```python
from build123d import *

# Parameters (mm, degrees)
BOSS_EXTRUDE1_START     = -38.1
SKETCH1_R               = 14.2875
SKETCH1_R_2             = 3.175
SKETCH1_R_3             = 3.2639
BOSS_EXTRUDE1_DEPTH     = 9.525
CUT_EXTRUDE1_REACH      = 194.229
CUT_EXTRUDE1_END_RADIUS = 14.2875
SKETCH2_R               = 2.6035
FILLET1_R               = 6.35


with BuildPart() as part:
    # Sketch1 → Boss-Extrude1 (new body)
    with BuildSketch(Plane(origin=(0, 0, 0), x_dir=(0, 0, -1), z_dir=(1, 0, 0)).offset(BOSS_EXTRUDE1_START)):
        with BuildLine():
            Line((-42.525623825, 632.652514423), (-55.415953018, 737.356140976))
            Line((-55.415953018, 737.356140976), (-55.415953018, 788.156140976))
            Line((-55.415953018, 788.156140976), (20.784046982, 788.156140976))
            Line((20.784046982, 788.156140976), (20.784046982, 737.356140976))
            Line((20.784046982, 737.356140976), (7.89371779, 632.652514423))
            ThreePointArc((7.89371779, 632.652514423), (-17.315953018, 610.356140976), (-42.525623825, 632.652514423))
        make_face()
        with Locations((-17.315953018, 635.756140976)):
            Circle(SKETCH1_R, mode=Mode.SUBTRACT)
        with Locations((-45.890953018, 775.456140976)):
            Circle(SKETCH1_R_2, mode=Mode.SUBTRACT)
        with Locations((-17.315953018, 762.756140976)):
            Circle(SKETCH1_R_2, mode=Mode.SUBTRACT)
        with Locations((-45.890953018, 750.056140976)):
            Circle(SKETCH1_R_2, mode=Mode.SUBTRACT)
        with Locations((11.259046982, 750.056140976)):
            Circle(SKETCH1_R_2, mode=Mode.SUBTRACT)
        with Locations((11.259046982, 775.456140976)):
            Circle(SKETCH1_R_2, mode=Mode.SUBTRACT)
        with Locations((8.084046982, 696.081140976)):
            Circle(SKETCH1_R_3, mode=Mode.SUBTRACT)
        with Locations((-17.315953018, 680.206140976)):
            Circle(SKETCH1_R_2, mode=Mode.SUBTRACT)
        with Locations((-42.715953018, 696.081140976)):
            Circle(SKETCH1_R_3, mode=Mode.SUBTRACT)
    extrude(amount=-BOSS_EXTRUDE1_DEPTH)

    # Cut-Extrude1: up to this cylinder (the profile starts outside it)
    cut_extrude1_end = Plane(origin=(-42.8625, 635.756140976, 17.315953018), z_dir=(1, 0, 0)) * Cylinder(CUT_EXTRUDE1_END_RADIUS, 418.033, mode=Mode.PRIVATE)
    # Sketch2 → Cut-Extrude1 (cut, up to the surface)
    with BuildSketch(Plane(origin=(0, 610.356140976, 0), x_dir=(-1, 0, 0), z_dir=(0, -1, 0)), mode=Mode.PRIVATE) as cut_extrude1_sk1:
        with Locations(Location((42.8625, -17.315953018, 0), (0, 0, 90))):
            Circle(SKETCH2_R)
    cut_extrude1_tool1 = extrude(cut_extrude1_sk1.sketch, amount=-CUT_EXTRUDE1_REACH, mode=Mode.PRIVATE) - cut_extrude1_end
    add(cut_extrude1_tool1.solids().sort_by_distance((-42.8625, 610.356141, 17.315953))[0], mode=Mode.SUBTRACT)

    # Fillet1
    fillet1_edges = [part.edges().sort_by_distance(p)[0] for p in [
        (-42.8625, 737.356140976, 55.415953018),
        (-42.8625, 788.156140976, 55.415953018),
        (-42.8625, 788.156140976, -20.784046982),
        (-42.8625, 737.356140976, -20.784046982),
    ]]
    fillet(fillet1_edges, radius=FILLET1_R)


solid = part.part
```
The model under review builds one solid part; all positions refer to its coordinate system, in mm. Give positions to 0.01 mm unless a question says otherwise; leave off trailing zeros. Write each loop counter-clockwise with the first axis right and the second up, starting at its lowest first coordinate (ties: lowest second). Pieces come first, ordered by that corner, then holes. Notation, with made-up numbers: (-4, -7.5) -> (29, -7.5) arc R31 cw to (29, 16.5) -> close; hole circle Ø2 at (34, 3.25). An arc over 180 degrees is marked (long way). Put each result on its own line as item: value.
(1) For pin 1 Ø8.5 at (y, z) = (775.46, 45.89) entering from +X; pin 2 Ø2 at (x, y) = (-42.5, 686.5) entering from -Z, all flat-tipped, find the tip position at first contact; note any pin that passes through.
Results are:
pin 1: x = -38.1
pin 2: z = -14.65
(2) We need section B-B, the plane z = 27. Give the boundary of the cut face in (x, y) (3 decimals).
Results are:
outline: (-47.625, 612.275) -> (-38.1, 612.275) -> (-38.1, 625.251) -> (-47.625, 625.251) -> close; (-47.625, 646.261) -> (-38.1, 646.261) -> (-38.1, 788.156) -> (-47.625, 788.156) -> close
(3) We need section C-C, the plane y = 729.5. Give the boundary of the cut face in (x, z) (3 decimals), and give its area (3 significant figures).
Results are:
outline: (-47.625, -19.817) -> (-38.1, -19.817) -> (-38.1, 54.449) -> (-47.625, 54.449) -> close
area: 707 mm²
(4) We need section A-A, the plane z = 10. Give the boundary of the cut face in (x, y) (3 decimals), and give its area (3 significant figures).
Results are:
outline: (-47.625, 611.433) -> (-38.1, 611.433) -> (-38.1, 623.484) -> (-47.625, 623.484) -> close; (-47.625, 648.028) -> (-38.1, 648.028) -> (-38.1, 788.156) -> (-47.625, 788.156) -> close
area: 1,450 mm²
(5) We need section D-D, the plane z = -0.5. Give the boundary of the cut face in (x, y) (3 decimals).
Results are:
outline: (-47.625, 617.652) -> (-38.1, 617.652) -> (-38.1, 788.156) -> (-47.625, 788.156) -> close
(6) To check wall thickness, follow probe 1 along Z at (x, y) = (-42.25, 696); probe 2 along Z at (x, y) = (-43.75, 697); probe 3 along Y at (x, z) = (-46.5, 18.5). State the ranges of each line that lie inside material, in increasing order. Write a range as from..to.
Results are:
probe 1: -15.69..-11.35, -4.82..39.45, 45.98..50.32
probe 2: -15.82..-11.22, -4.95..39.58, 45.85..50.45
probe 3: 610.38..621.52, 649.99..677.26, 683.15..759.81, 765.7..788.16
(7) The part is to be moulded in two halves that separate along Y. For faces 1 (the cylindrical face through (-45.17, 615.95, 16.11)), 2 (the cylindrical face through (-42.93, 786.25, -18.97)), 3 (the cylindrical face through (-42.796, 748.124, -8.739)), 4 (the flat face through (-42.8, 685.5, -14.4)), say which applies: pulls with the +Y half, pulls with the -Y half, needs draft (parallel to the pull), parting line crosses it, or undercut.
Results are:
face 1: needs draft
face 2: pulls with the +Y half
face 3: undercut
face 4: pulls with the -Y half
